from build123d import *

# Parameters (mm, degrees)
SKETCH1_R           = 2
BOSS_EXTRUDE1_DEPTH = 2
SKETCH1_3_R         = 6
BOSS_EXTRUDE2_DEPTH = 3.5
CUT_EXTRUDE2_DEPTH  = 10
SKETCH2_R           = 1.4
BOSS_EXTRUDE4_DEPTH = 3.5
FILLET3_R           = 1


with BuildPart() as part:
    # Sketch1 → Boss-Extrude1 (new body)
    with BuildSketch(Plane(origin=(0, 0, 0), x_dir=(1, 0, 0), z_dir=(0, 1, 0))):
        with BuildLine():
            Line((-52.5, -49), (52.5, -49))
            ThreePointArc((52.5, -49), (59.571067812, -46.071067812), (62.5, -39))
            Line((62.5, -39), (62.5, 39))
            ThreePointArc((62.5, 39), (59.571067812, 46.071067812), (52.5, 49))
            Line((52.5, 49), (-52.5, 49))
            ThreePointArc((-52.5, 49), (-59.571067812, 46.071067812), (-62.5, 39))
            Line((-62.5, 39), (-62.5, -39))
            ThreePointArc((-62.5, -39), (-59.571067812, -46.071067812), (-52.5, -49))
        make_face()
        with Locations(Location((53.5, 40, 0), (0, 0, 270))):
            Circle(SKETCH1_R, mode=Mode.SUBTRACT)
        with Locations(Location((-53.5, 40, 0), (0, 0, 270))):
            Circle(SKETCH1_R, mode=Mode.SUBTRACT)
        with Locations(Location((53.5, -40, 0), (0, 0, 270))):
            Circle(SKETCH1_R, mode=Mode.SUBTRACT)
        with Locations(Location((-53.5, -40, 0), (0, 0, 270))):
            Circle(SKETCH1_R, mode=Mode.SUBTRACT)
    extrude(amount=BOSS_EXTRUDE1_DEPTH)

    # Sketch1_3 → Boss-Extrude2 (add)
    # profile 1 of 4: a face of its own
    with BuildSketch(Plane(origin=(0, 0, 0), x_dir=(1, 0, 0), z_dir=(0, 1, 0))):
        with Locations(Location((53.5, 40, 0), (0, 0, 270))):
            Circle(SKETCH1_3_R)
        Polygon((57.968015998, 40.535567959), (55.270192541, 44.137199339), (50.802176543, 43.601631379), (49.031984002, 39.464432041), (51.729807459, 35.862800661), (56.197823457, 36.398368621), align=None, mode=Mode.SUBTRACT)
    # profile 2 of 4: a face of its own
    with BuildSketch(Plane(origin=(0, 0, 0), x_dir=(1, 0, 0), z_dir=(0, 1, 0))):
        with Locations(Location((-53.5, 40, 0), (0, 0, 270))):
            Circle(SKETCH1_3_R)
        Polygon((-49.031984002, 40.535567959), (-51.729807459, 44.137199339), (-56.197823457, 43.601631379), (-57.968015998, 39.464432041), (-55.270192541, 35.862800661), (-50.802176543, 36.398368621), align=None, mode=Mode.SUBTRACT)
    # profile 3 of 4: a face of its own
    with BuildSketch(Plane(origin=(0, 0, 0), x_dir=(1, 0, 0), z_dir=(0, 1, 0))):
        with Locations(Location((53.5, -40, 0), (0, 0, 270))):
            Circle(SKETCH1_3_R)
        Polygon((57.968015998, -39.464432041), (55.270192541, -35.862800661), (50.802176543, -36.398368621), (49.031984002, -40.535567959), (51.729807459, -44.137199339), (56.197823457, -43.601631379), align=None, mode=Mode.SUBTRACT)
    # profile 4 of 4: a face of its own
    with BuildSketch(Plane(origin=(0, 0, 0), x_dir=(1, 0, 0), z_dir=(0, 1, 0))):
        with Locations(Location((-53.5, -40, 0), (0, 0, 270))):
            Circle(SKETCH1_3_R)
        Polygon((-49.031984002, -39.464432041), (-51.729807459, -35.862800661), (-56.197823457, -36.398368621), (-57.968015998, -40.535567959), (-55.270192541, -44.137199339), (-50.802176543, -43.601631379), align=None, mode=Mode.SUBTRACT)
    extrude(amount=-BOSS_EXTRUDE2_DEPTH)

    # Sketch2_4 → Cut-Extrude2 (cut)
    with BuildSketch(Plane(origin=(0, 0, 0), x_dir=(1, 0, 0), z_dir=(0, 1, 0))):
        with BuildLine():
            ThreePointArc((13.453203488, 8.809870368), (9.040022455, 0), (13.453203488, -8.809870368))
            Line((13.453203488, -8.809870368), (34.913181033, -24.854713392))
            ThreePointArc((34.913181033, -24.854713392), (46.426712462, -25.879857224), (52.5, -16.044843024))
            Line((52.5, -16.044843024), (52.5, 16.044843024))
            ThreePointArc((52.5, 16.044843024), (46.426712462, 25.879857224), (34.913181033, 24.854713392))
            Line((34.913181033, 24.854713392), (13.453203488, 8.809870368))
        make_face()
        with BuildLine():
            Line((-2.994008621, 12.227307358), (-28.096484295, 30.995513469))
            ThreePointArc((-28.096484295, 30.995513469), (-29.847074321, 36.577587929), (-25.102475674, 40))
            Line((-25.102475674, 40), (25.102475674, 40))
            ThreePointArc((25.102475674, 40), (29.847074321, 36.577587929), (28.096484295, 30.995513469))
            Line((28.096484295, 30.995513469), (2.994008621, 12.227307358))
            ThreePointArc((2.994008621, 12.227307358), (0, 11.231793889), (-2.994008621, 12.227307358))
        make_face()
        with BuildLine():
            ThreePointArc((-34.913181033, 24.854713392), (-46.426712462, 25.879857224), (-52.5, 16.044843024))
            Line((-52.5, 16.044843024), (-52.5, -16.044843024))
            ThreePointArc((-52.5, -16.044843024), (-46.426712462, -25.879857224), (-34.913181033, -24.854713392))
            Line((-34.913181033, -24.854713392), (-13.453203488, -8.809870368))
            ThreePointArc((-13.453203488, -8.809870368), (-9.040022455, 0), (-13.453203488, 8.809870368))
            Line((-13.453203488, 8.809870368), (-34.913181033, 24.854713392))
        make_face()
        with BuildLine():
            Line((-25.102475674, -40), (25.102475674, -40))
            ThreePointArc((25.102475674, -40), (29.847074321, -36.577587929), (28.096484295, -30.995513469))
            Line((28.096484295, -30.995513469), (2.994008621, -12.227307358))
            ThreePointArc((2.994008621, -12.227307358), (0, -11.231793889), (-2.994008621, -12.227307358))
            Line((-2.994008621, -12.227307358), (-28.096484295, -30.995513469))
            ThreePointArc((-28.096484295, -30.995513469), (-29.847074321, -36.577587929), (-25.102475674, -40))
        make_face()
    extrude(amount=CUT_EXTRUDE2_DEPTH, mode=Mode.SUBTRACT)

    # Sketch2 → Boss-Extrude4 (add)
    with BuildSketch(Plane(origin=(0, 0, 0), x_dir=(1, 0, 0), z_dir=(0, 1, 0))):
        with Locations(Location((17.5, 17.5, 0), (0, 0, 90))):
            Circle(SKETCH2_R)
        with Locations(Location((-17.5, -17.5, 0), (0, 0, 90))):
            Circle(SKETCH2_R)
        with Locations(Location((17.5, -17.5, 0), (0, 0, 90))):
            Circle(SKETCH2_R)
        with Locations(Location((-17.5, 17.5, 0), (0, 0, 270))):
            Circle(SKETCH2_R)
    extrude(amount=-BOSS_EXTRUDE4_DEPTH)

    # Fillet3
    fillet3_edges = [part.edges().sort_by_distance(p)[0] for p in [
        (17.5, 0, -16.1),
        (-17.5, 0, 18.9),
        (17.5, 0, 18.9),
        (-17.5, 0, -18.9),
    ]]
    fillet(fillet3_edges, radius=FILLET3_R)


solid = part.part
For this review, take the finished solid that the model builds, in its own axes (mm). A direction names the side the tool comes from. Round coordinates to 2 decimals unless told otherwise and drop trailing zeros. Loops run counter-clockwise (first coordinate to the right, second up) from the corner with the lowest first, then second, coordinate; pieces in that order, holes last. Notation, with made-up numbers: (-33.5, 9) - (5.5, 9) arc R22 ccw to (5.5, 44) - close; hole circle Ø8 at (38, 16.25). An arc over 180 degrees is marked (long way). One line per item, written item: value. Start each with the question number.
Item 1: Clearance check with flat-ended pins moving along their axes: pin 1 Ø4 at (x, z) = (54.5, -41) entering from -Y; pin 2 Ø3 at (x, z) = (-53.5, 40) entering from +Y. State where each tip first meets the part, or that it passes through.
Item 2: Take a section at C-C (x = -5). Give the boundary of the cut face in (y, z), plus the area to 3 significant figures.
Item 3: The part is to be moulded in two halves that separate along X. For faces 1 (the cylindrical face through (-52.148, 0.986, 38.526)), 2 (the flat face through (55, -3.5, -36)), 3 (the cylindrical face through (-59.49, 0.99, -46.15)), 4 (the flat face through (-56.64, -1.73, -37.69)), say which applies: +X half, -X half, draft (parallel to the pull), parting line (faces both ways), or undercut.
Item 4: Take a section at A-A (z = 32.5). Give the boundary of the cut face in (x, y).
Item 5: For faces 5 (the flat face through (17, -3.5, -17)), 6 (the flat face through (-53.933, -1.726, 36.127)), 7 (the cylindrical face through (9.04, 0.99, -0.14)), list the 3-axis set-ups (+Z, -Z, +X, -X, +Y, -Y) from which the entire face can be reached by the end or side of a thin tool; tool diameter is ignored.
Item 6: Take a section at D-D (z = 17.5). Give the boundary of the cut face in (x, y).
Item 7: Take a section at B-B (x = -17.5). Give the boundary of the cut face in (y, z), plus the area to 3 significant figures.
Item 8: For L1, parallel to X at y = 0.5, z = -0.5; L2, parallel to X at y = 1.55, z = -13; L3, parallel to Z at x = -19, y = 1.5, list the stretches that pass through material, from the lowest coordinate up.
Answer below:
1. pin 1: stops at y = 0
1. pin 2: passes through
2. outline: (0, -49) - (2, -49) - (2, -40) - (0, -40) - close; (0, -13.73) - (2, -13.73) - (2, 13.73) - (0, 13.73) - close; (0, 40) - (2, 40) - (2, 49) - (0, 49) - close
2. area: 90.9 mm2
3. face 1: undercut
3. face 2: draft
3. face 3: -X half
3. face 4: undercut
4. outline: (-62.5, 0) - (-29.43, 0) - (-29.43, 2) - (-62.5, 2) - close; (29.43, 0) - (62.5, 0) - (62.5, 2) - (29.43, 2) - close
5. face 5: +Z, -Z, +X, -X, -Y
5. face 6: -Y
5. face 7: +Y, -Y
6. outline: (-62.5, 0) - (-52.4, 0) - (-52.4, 2) - (-62.5, 2) - close; (-25.08, 0) - (-19.9, 0) arc R1 cw to (-18.9, -1) - (-18.9, -3.5) - (-16.1, -3.5) - (-16.1, -1) arc R1 cw to (-15.1, 0) - (-10.05, 0) - (-10.05, 2) - (-25.08, 2) - close; (10.05, 0) - (15.1, 0) arc R1 cw to (16.1, -1) - (16.1, -3.5) - (18.9, -3.5) - (18.9, -1) arc R1 cw to (19.9, 0) - (25.08, 0) - (25.08, 2) - (10.05, 2) - close; (52.4, 0) - (62.5, 0) - (62.5, 2) - (52.4, 2) - close
7. outline: (-3.5, -18.9) - (-1, -18.9) arc R1 cw to (0, -19.9) - (0, -23.07) - (2, -23.07) - (2, -11.84) - (0, -11.84) - (0, -15.1) arc R1 cw to (-1, -16.1) - (-3.5, -16.1) - close; (-3.5, 16.1) - (-1, 16.1) arc R1 cw to (0, 15.1) - (0, 11.84) - (2, 11.84) - (2, 23.07) - (0, 23.07) - (0, 19.9) arc R1 cw to (-1, 18.9) - (-3.5, 18.9) - close; (0, -49) - (2, -49) - (2, -40) - (0, -40) - close; (0, 40) - (2, 40) - (2, 49) - (0, 49) - close
7. area: 101 mm2
8. L1: x = -62.5 to -52.5, -9.05 to 9.05, 52.5 to 62.5
8. L2: x = -62.5 to -52.5, -19.06 to -4.03, 4.03 to 19.06, 52.5 to 62.5
8. L3: z = -49 to -40, -24.19 to -12.96, 12.96 to 24.19, 40 to 49
